Design review of the part built by this model. Coordinates are the model's own, in mm. A direction names the side the tool comes from. Coordinates: 2 decimals unless noted, no trailing zeros. Order: outer loops, then holes, each group sorted by start corner. A loop starts at its lowest first (then second) coordinate and runs counter-clockwise, first axis right, second up. Notation, with made-up numbers: (81.25, -26) -> (108.25, -26) arc R23 cw to (108.25, 2) -> close; hole circle Ø11 at (23.5, -27.75). An arc over 180 degrees is marked (long way). Write item = value, one per line.
```python
from build123d import *

# Parameters (mm, degrees)
F0_W     = 124.741532
F0_H     = 89.657984
F1_DEPTH = 41.402
F2_R     = 33.425555
F3_DEPTH = 34.798
F4_R     = 30.303801
F5_DEPTH = 96.266


with BuildPart() as f1:
    # F0 (on Front) → F1 (new body)
    with BuildSketch(Plane.XZ):
        Rectangle(F0_W, F0_H)
    extrude(amount=F1_DEPTH)

    # F2 (on face) → F3 (join)
    with BuildSketch(Plane.XZ.offset(41.402)):
        Circle(F2_R)
    extrude(amount=F3_DEPTH)

    # F4 (on face) → F5 (cut)
    with BuildSketch(Plane.XZ.offset(76.2)):
        Circle(F4_R)
    extrude(amount=-F5_DEPTH, mode=Mode.SUBTRACT)


solid = f1.part
```
(1) We need section A-A (x = 0). Write out the cut boundary in (y, z).
Report:
outline = (-76.2, -33.43) -> (-41.4, -33.43) -> (-41.4, -44.83) -> (0, -44.83) -> (0, -30.3) -> (-76.2, -30.3) -> close; (-76.2, 30.3) -> (0, 30.3) -> (0, 44.83) -> (-41.4, 44.83) -> (-41.4, 33.43) -> (-76.2, 33.43) -> close
(2) The part is to be moulded in two halves that separate along Z. For faces 1 (the flat face through (7, -76.2, -30)), 2 (the cylindrical face through (-6.569, -38.633, -29.583)), 3 (the cylindrical face through (-4.35, -58.56, 33.14)), say which applies: released by +Z, released by -Z, zero draft, split by the parting line, or undercut.
Report:
face_1 = zero draft
face_2 = undercut
face_3 = split by the parting line
(3) We need section B-B (z = 0). Write out the cut boundary in (x, y), and give its area (3 significant figures).
Report:
outline = (-62.37, -41.4) -> (-33.43, -41.4) -> (-33.43, -76.2) -> (-30.3, -76.2) -> (-30.3, 0) -> (-62.37, 0) -> close; (30.3, -76.2) -> (33.43, -76.2) -> (33.43, -41.4) -> (62.37, -41.4) -> (62.37, 0) -> (30.3, 0) -> close
area = 2,870 mm²
(4) For L1, parallel to Z at x = 0.5, y = -52.5; L2, parallel to Y at x = -32, z = -32; L3, parallel to Z at x = 0, y = -25, list the stretches that pass through material, from the lowest coordinate up.
Report:
L1 = -33.42 to -30.3, 30.3 to 33.42
L2 = -41.4 to 0
L3 = -44.83 to -30.3, 30.3 to 44.83
(5) We need section D-D (x = 38.5). Write out the cut boundary in (y, z), and give its area (3 significant figures).
Report:
outline = (-41.4, -44.83) -> (0, -44.83) -> (0, 44.83) -> (-41.4, 44.83) -> close
area = 3,710 mm²
(6) We need section C-C (y = -55.5). Write out the cut boundary in (x, z).
Report:
outline = circle Ø66.85 at (0, 0); hole circle Ø60.61 at (0, 0)
(7) Insertion check: pin 1 (5 mm diameter, centred on y = -53, z = -10.5, fed in from +X). The pin has a flat end and moves straight along its axis. Give the tip position at first contact, or say it passes through.
Report:
pin_1 = 32.45
(8) For faces 4 (the flat face through (-15, -41.402, 31)), 5 (the flat face through (-1, -20, -44.829)), list the 3-axis set-ups (+Z, -Z, +X, -X, +Y, -Y) from which the entire face can be reached by the end or side of a thin tool; tool diameter is ignored.
Report:
face_4 = -Y
face_5 = -Z, +X, -X, +Y, -Y
